Read the model definition and answer for the solid it produces. Units are mm, in the model's axes. Give positions to 0.01 mm unless a question says otherwise; leave off trailing zeros. Loops run counter-clockwise (first coordinate to the right, second up) from the corner with the lowest first, then second, coordinate; pieces in that order, holes last.
(1) Find section B-B, the plane z = -58. Write down the section's boundary in (x, y).
(2) Find section D-D, the plane y = 64. Write down the section's boundary in (x, z).
(3) Find section C-C, the plane z = -18. Write down the section's boundary in (x, y).
(4) Find section A-A, the plane x = 249.5. Write down the section's boundary in (y, z).
(5) Straight lines are drawn through the part: probe 1 along Z at (x, y) = (819.5, 10); probe 2 along Z at (x, y) = (948.5, -2); probe 3 along Y at (x, z) = (410.5, -59). For each, find the intervals that lie inside material, in ascending order.
(6) Each of these flat-tipped pins is pushed along its axis until it touches: P1, Ø1.5, axis at x = 486, z = -53, coming from the +Y side; P2, Ø5, axis at x = 318.5, z = 49.5, coming from the +Y side; P3, Ø4, axis at x = 154, z = -7.5, coming from the -Y side. Where does it stop, or does it pass through?
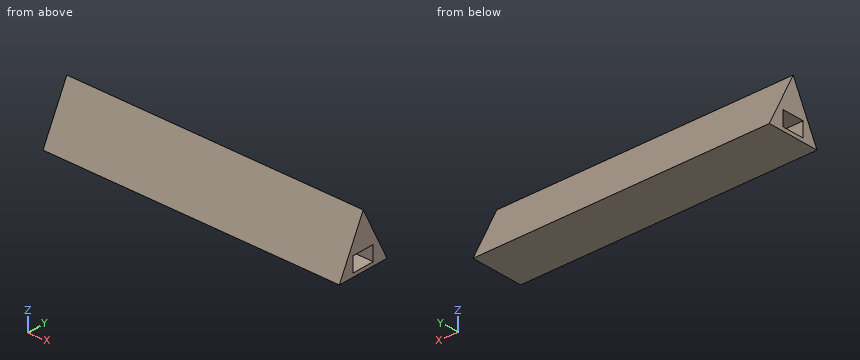
```python
from build123d import *

# Parameters (mm, degrees)
F0_W     = 76.2
F0_H     = 50.8
F1_DEPTH = 1016


with BuildPart() as f1:
    # F0 (on Right) → F1 (new body)
    with BuildSketch(Plane.YZ):
        Polygon((0, 91.370057), (-90.625222, -90.625168), (90.376866, -90.625168), align=None)
        with Locations((0, -52.525168)):
            Rectangle(F0_W, F0_H, mode=Mode.SUBTRACT)
    extrude(amount=F1_DEPTH)


solid = f1.part
```
Entries:
1. outline: (0, -74.38) - (1016, -74.38) - (1016, -38.1) - (0, -38.1) - close; (0, 38.1) - (1016, 38.1) - (1016, 74.18) - (0, 74.18) - close
2. outline: (0, -90.63) - (1016, -90.63) - (1016, -37.51) - (0, -37.51) - close
3. outline: (0, -54.46) - (1016, -54.46) - (1016, 54.31) - (0, 54.31) - close
4. outline: (-90.63, -90.63) - (90.38, -90.63) - (0, 91.37) - close; hole (-38.1, -77.93) - (38.1, -77.93) - (38.1, -27.13) - (-38.1, -27.13) - close
5. probe 1: z = -90.63 to -77.93, -27.13 to 71.23
5. probe 2: z = -90.63 to -77.93, -27.13 to 87.35
5. probe 3: y = -74.88 to -38.1, 38.1 to 74.67
6. P1: stops at y = 72.07
6. P2: stops at y = 22.03
6. P3: stops at y = -50.23
